Build history of the part. All positions in model axes, mm. A direction names the side the tool comes from. Give positions to 0.01 mm unless a question says otherwise; leave off trailing zeros. Loops run counter-clockwise (first coordinate to the right, second up) from the corner with the lowest first, then second, coordinate; pieces in that order, holes last. Notation, with made-up numbers: (-8, 78.25) -> (13, 78.25) arc R24 ccw to (13, 99.25) -> close; hole circle Ø7 at (13, 71.5). An arc over 180 degrees is marked (long way). Answer as a JSON object with one key per item and string values. Group by question number.
from build123d import *

# Parameters (mm, degrees)
SALIENTE_EXTRUIR1_DEPTH = 3
CORTAR_EXTRUIR1_REACH   = 102.701
CROQUIS2_R              = 1.2
CORTAR_EXTRUIR2_REACH   = 99.382
CROQUIS3_R              = 1.2
SALIENTE_EXTRUIR2_DEPTH = 6
CORTAR_EXTRUIR3_REACH   = 94.93
CROQUIS5_R              = 1.2


with BuildPart() as part:
    # Croquis1 → Saliente-Extruir1 (new, symmetric)
    with BuildSketch(Plane.XY):
        Polygon((36.601721277, 88.42375405), (39.249173289, 87.512163218), (37.360877993, 82.028155479), (45.422960067, 5.322568365), (50.680147873, 5.322568365), (50.680147873, 2.522568365), (42.685021257, 2.243372391), (34.322744196, 81.805124021), align=None)
    extrude(amount=SALIENTE_EXTRUIR1_DEPTH, both=True)

    # Croquis2 → Cortar-Extruir1 (cut, up to next)
    with BuildSketch(Plane(origin=(8.150038197, -2.806283201, 0), x_dir=(0, 0, -1), z_dir=(0.9455185755993173, -0.3255681544571552, 0)), mode=Mode.PRIVATE) as cortar_extruir1_sk1:
        with Locations(Location((0, 92.622656825, 0), (0, 0, 90))):
            Circle(CROQUIS2_R)
    cortar_extruir1_tool1 = extrude(cortar_extruir1_sk1.sketch, amount=-CORTAR_EXTRUIR1_REACH, mode=Mode.PRIVATE) & part.part
    add(cortar_extruir1_tool1.solids().sort_by_distance((38.305026, 84.770159, 0))[0], mode=Mode.SUBTRACT)

    # Cortar-Extruir2: up to this plane
    cortar_extruir2_end = Plane(origin=(42.685021257, 2.243372391, 3), z_dir=(-0.03489949670250159, 0.9993908270190958, 0))
    # Croquis3 → Cortar-Extruir2 (cut, up to the surface)
    with BuildSketch(Plane(origin=(0, 5.322568365, 0), x_dir=(1, 0, 0), z_dir=(0, 1, 0)), mode=Mode.PRIVATE) as cortar_extruir2_sk1:
        with Locations(Location((48.05155397, 0, 0), (0, 0, 180))):
            Circle(CROQUIS3_R)
    cortar_extruir2_tool1 = split(extrude(cortar_extruir2_sk1.sketch, amount=-CORTAR_EXTRUIR2_REACH, mode=Mode.PRIVATE), bisect_by=cortar_extruir2_end, keep=Keep.BOTH, mode=Mode.PRIVATE)
    add(cortar_extruir2_tool1.solids().sort_by_distance((48.051554, 5.322568, 0))[0], mode=Mode.SUBTRACT)

    # Croquis4 → Saliente-Extruir2 (add)
    with BuildSketch(Plane.XY.offset(3)):
        Polygon((36.601721277, 88.42375405), (37.610982556, 91.354861634), (48.957205463, 87.448043781), (47.947944184, 84.516936196), align=None)
    extrude(amount=-SALIENTE_EXTRUIR2_DEPTH)

    # Croquis5 → Cortar-Extruir3 (cut, up to next)
    with BuildSketch(Plane(origin=(32.10839637, 93.249554003, 0), x_dir=(0.9455185755993183, -0.3255681544571526, 0), z_dir=(0.3255681544571526, 0.9455185755993183, 0)), mode=Mode.PRIVATE) as cortar_extruir3_sk1:
        with Locations(Location((13.95964895, 0, 0), (0, 0, 180))):
            Circle(CROQUIS5_R)
    cortar_extruir3_tool1 = extrude(cortar_extruir3_sk1.sketch, amount=-CORTAR_EXTRUIR3_REACH, mode=Mode.PRIVATE) & part.part
    add(cortar_extruir3_tool1.solids().sort_by_distance((45.307504, 88.704737, 0))[0], mode=Mode.SUBTRACT)


solid = part.part
(1) Pin check, flat tips, straight feed: pin 1 (1 mm diameter, centred on y = 72.5, z = -1, fed in from +X); pin 2 (1 mm diameter, centred on y = 38, z = -2, fed in from -X); pin 3 (1.5 mm diameter, centred on y = 46.5, z = -2, fed in from -X); pin 4 (2 mm diameter, centred on x = 44.5, y = 37, fed in from +Z). Stop position of each tip, or through.
(2) Saw through at A-A on z = 0. List the corners of the cut face in (x, y).
(3) Probe line 1 along Y through (x, z) = (46.5, -0.9); line 2 along X through (y, z) = (3.35, 0); line 3 along X through (y, z) = (4.35, 0). List the from-to ranges inside material, lowest first. Write a range as [from, to].
(4) 3-axis set-ups, long thin cutter, end or side, ignore diameter. For faces 1 (the flat face through (38.32, 84.81, 1.38)), 2 (the flat face through (50.68, 4, 0)), 3 (the cylindrical face through (43.728, 87.632, 0.36)), 4 (the flat face through (47, 5.323, 1)), 5 (the cylindrical face through (46.943, 3.876, -0.46)): which of +Z, -Z, +X, -X, +Y, -Y reach the whole face in a straight line?
(5) Saw through at B-B on y = 67. List the corners of the cut face in (x, z), plus the area to 3 significant figures.
(6) Pull direction Z, two halves, no side cores. Call faces 6 (the flat face through (40, 50, 3)), 7 (the cylindrical face through (36.61, 84.086, 0.053)), 8 (the flat face through (38.562, 41.467, 0.042)), 9 (the flat face through (40, 50, -3)): pulls with the +Z half, pulls with the -Z half, needs draft (parallel to the pull), parting line crosses it, or undercut.
Calculated:
{
 "1": {"pin 1": "stops at x = 38.41", "pin 2": "stops at x = 38.87", "pin 3": "stops at x = 37.95", "pin 4": "passes through"},
 "2": {"outline": "(34.32, 81.81) -> (42.69, 2.24) -> (46.85, 2.39) -> (46.85, 5.32) -> (45.42, 5.32) -> (37.36, 82.03) -> (37.91, 83.64) -> (35.27, 84.55) -> close; (36.05, 86.82) -> (38.7, 85.9) -> (39.25, 87.51) -> (43.16, 86.16) -> (44.17, 89.1) -> (37.61, 91.35) -> close; (45.43, 85.38) -> (47.95, 84.52) -> (48.96, 87.45) -> (46.44, 88.31) -> close; (49.25, 2.47) -> (50.68, 2.52) -> (50.68, 5.32) -> (49.25, 5.32) -> close"},
 "3": {"line 1": "y = [2.38, 5.32], [85.02, 88.29]", "line 2": "x = [42.57, 46.85], [49.25, 50.68]", "line 3": "x = [42.46, 46.85], [49.25, 50.68]"},
 "4": {"face 1": "+Z, -Z", "face 2": "+Z, -Z, +X, +Y, -Y", "face 3": "none", "face 4": "+Z, -Z, +X", "face 5": "-Y"},
 "5": {"outline": "(35.88, -3) -> (38.94, -3) -> (38.94, 3) -> (35.88, 3) -> close", "area": "18.4 mm^2"},
 "6": {"face 6": "pulls with the +Z half", "face 7": "undercut", "face 8": "needs draft", "face 9": "pulls with the -Z half"}
}
